Read the model definition and answer for the solid it produces. Units are mm, in the model's axes. Round coordinates to 2 decimals unless told otherwise and drop trailing zeros. Order: outer loops, then holes, each group sorted by start corner. A loop starts at its lowest first (then second) coordinate and runs counter-clockwise, first axis right, second up. Notation, with made-up numbers: (4, -7.5) - (18, -7.5) arc R18 cw to (18, 11.5) - close; hole circle Ø4 at (15, -15). An arc over 180 degrees is marked (long way). Answer as a JSON object with one key per item and string values. Group by question number.
Q1. A cutting plane is placed at A-A on y = -37.5. Determine the outline of the cut face in (x, z).
Q2. A cutting plane is placed at C-C on x = -3. Determine the outline of the cut face in (y, z).
Q3. Consider line 1 (Y direction, x = -3, z = 1); line 2 (Y direction, x = -6.5, z = 4.2); line 3 (X direction, y = -40, z = 2.35). Determine where each line is inside the solid, lowest interval first.
Q4. A cutting plane is placed at B-B on z = 2.45. Determine the outline of the cut face in (x, y).
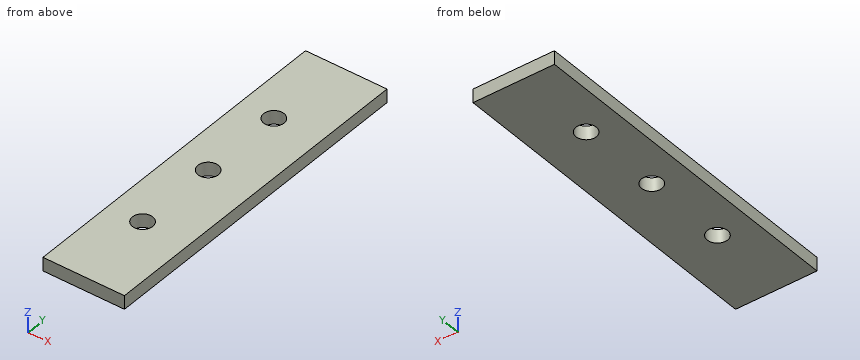
```python
from build123d import *

# Parameters (mm, degrees)
SKETCH1_W            = 36
SKETCH1_H            = 150
BOSS_EXTRUDE1_DEPTH  = 6
M8_CLEARANCE_HOLE1_D = 9


with BuildPart() as part:
    # Sketch1 → Boss-Extrude1 (new body)
    with BuildSketch(Plane.XY):
        Rectangle(SKETCH1_W, SKETCH1_H)
    extrude(amount=BOSS_EXTRUDE1_DEPTH)

    # M8 Clearance Hole1 (through all)
    with Locations(Plane.XY.offset(6)):
        with Locations((-3, 37.5), (-3, 0), (-3, -37.5)):
            Hole(M8_CLEARANCE_HOLE1_D / 2)


solid = part.part
```
Result set:
{
 "1": {"outline": "(-18, 0) - (-7.5, 0) - (-7.5, 6) - (-18, 6) - close; (1.5, 0) - (18, 0) - (18, 6) - (1.5, 6) - close"},
 "2": {"outline": "(-75, 0) - (-42, 0) - (-42, 6) - (-75, 6) - close; (-33, 0) - (-4.5, 0) - (-4.5, 6) - (-33, 6) - close; (4.5, 0) - (33, 0) - (33, 6) - (4.5, 6) - close; (42, 0) - (75, 0) - (75, 6) - (42, 6) - close"},
 "3": {"line 1": "y = -75 to -42, -33 to -4.5, 4.5 to 33, 42 to 75", "line 2": "y = -75 to -40.33, -34.67 to -2.83, 2.83 to 34.67, 40.33 to 75", "line 3": "x = -18 to -6.74, 0.74 to 18"},
 "4": {"outline": "(-18, -75) - (18, -75) - (18, 75) - (-18, 75) - close; hole circle Ø9 at (-3, -37.5); hole circle Ø9 at (-3, 0); hole circle Ø9 at (-3, 37.5)"}
}
